from build123d import *

# Parameters (mm, degrees)
F2_DEPTH  = 25.4
F3_R      = 248.0240216894
F4_DEPTH  = 2540
F5_W      = 119.7975315154
F5_H      = 181.1522692442
F5_W_2    = 320.4690925777
F5_H_2    = 205.2030339837
F5_W_3    = 6.3688382506
F5_W_4    = 172.1075996757
F6_DEPTH  = 25.4
F7_R      = 40.7896547179
F8_DEPTH  = 2565.401
F9_R      = 164.1580524022
F10_DEPTH = 2514.6


with BuildPart() as f2:
    # F1 (on face) → F2 (new body)
    with BuildSketch(Plane.XY):
        Polygon((-21.2495476007, -69.6708932519), (-21.2495476007, 53.5316392779), (0, 53.5316392779), (0, 76.628908515), (-80.3218334913, 76.628908515), (-80.3218334913, -69.6708932519), align=None)
        Polygon((0, 76.628908515), (0, 53.5316392779), (0, -69.6708932519), (74.5332688093, -69.6708932519), (74.5332688093, 76.628908515), align=None)
        Polygon((0, -69.6708932519), (-21.2495476007, -69.6708932519), (-80.3218334913, -69.6708932519), (-80.3218334913, -80.1510289311), (74.5332688093, -80.1510289311), (74.5332688093, -69.6708932519), align=None)
    extrude(amount=F2_DEPTH)

    # F3 (on Top) → F4 (join)
    with BuildSketch(Plane.XY):
        with Locations((-47.1228808165, 30.5453538895)):
            Circle(F3_R)
    extrude(amount=-F4_DEPTH)

    # F5 (on face) → F6 (join)
    with BuildSketch(Plane.XY):
        with Locations((36.0827576369, 215.6281396747)):
            Rectangle(F5_W, F5_H)
        with Locations((-184.0505544096, 215.6281396747)):
            Rectangle(F5_W_2, F5_H)
        with Locations((-184.0505544096, 22.4504880607)):
            Rectangle(F5_W_2, F5_H_2)
        with Locations((99.1659425199, 215.6281396747)):
            Rectangle(F5_W_3, F5_H)
        Polygon((95.9815233946, -80.1510289311), (-23.8160081208, -80.1510289311), (-23.8160081208, -285.3540629148), (102.3503616452, -285.3540629148), (102.3503616452, -80.1510289311), align=None)
        with Locations((-184.0505544096, -182.752545923)):
            Rectangle(F5_W_2, F5_H_2)
        with Locations((188.404161483, 215.6281396747)):
            Rectangle(F5_W_4, F5_H)
        with Locations((188.404161483, 22.4504880607)):
            Rectangle(F5_W_4, F5_H_2)
        with Locations((188.404161483, -182.752545923)):
            Rectangle(F5_W_4, F5_H_2)
    extrude(amount=F6_DEPTH)

    # F7 (on face) → F8 (cut, through all)
    with BuildSketch(Plane.XY.offset(25.4)):
        with Locations((-161.9917303324, 89.3510133028)):
            Circle(F7_R)
    extrude(amount=-F8_DEPTH, mode=Mode.SUBTRACT)

    # F9 (on face) → F10 (cut)
    with BuildSketch(Plane.XY.offset(25.4)):
        Circle(F9_R)
    extrude(amount=-F10_DEPTH, mode=Mode.SUBTRACT)


solid = f2.part
Can you work these out from the model? Positions are in its coordinate system, mm. A direction names the side the tool comes from. Coordinates: 2 decimals unless noted, no trailing zeros. Order: outer loops, then holes, each group sorted by start corner. A loop starts at its lowest first (then second) coordinate and runs counter-clockwise, first axis right, second up. Notation, with made-up numbers: (65.5, 46.5) - (115.5, 46.5) arc R34 cw to (115.5, 83.5) - close; hole circle Ø6 at (77.5, 72.25). An arc over 180 degrees is marked (long way). Answer as a JSON object with one key per item and string values. Group by question number.
Q1. Will these pins go through, and if not, where does the flat tip stop? P1, Ø1.5, axis at x = 124, z = -2064, coming from the -Y side; P2, Ø12, axis at x = -163, z = -1143.5, coming from the -Y side; P3, Ø4, axis at y = 66, z = -1816, coming from the -X side.
Q2. We'd pull the mould along X, two halves only. Please class faces 3 (the face through (98, -183, 0)), 4 (the face through (-202.742, 91.144, -1239.342)), 5 (the face through (189.448, 105.045, -1252.22)): +X half, -X half, draft (parallel to the pull), parting line (faces both ways), or undercut.
Q3. Imagine slicing it at D-D (x = -225). Please give me the cut outline in (y, z), and give its area (3 significant figures).
Q4. I need wall thicknesses on line 1 (X direction, y = 123.5, z = -190); line 2 (Z direction, x = 184, y = -159.5); line 3 (X direction, y = 150, z = -421). Which ranges of each line are inside material? Lowest first, please. Write a range as from..to.
Q5. Imagine slicing it at A-A (x = 130). Please give me the cut outline in (y, z).
Q6. On a 3-axis mill with a long thin cutter (end or side, diameter ignored), from which of +Z, -Z, +X, -X, +Y, -Y can I reach the whole of each face in a straight line? I mean faces 1 (the face through (-2, 2, -2489.2)), 2 (the face through (-51, 34, -2540)). Say none if no direction works.
Q7. Imagine slicing it at C-C (z = -2331). Please give me the cut outline in (x, y), and give its area (3 significant figures).
Q8. Imagine slicing it at B-B (y = 0). Please give me the cut outline in (x, z).
Determined:
{
 "1": {"P1": "stops at y = -149.7", "P2": "stops at y = -191.81", "P3": "stops at x = -292.88"},
 "2": {"face 3": "draft", "face 4": "undercut", "face 5": "parting line"},
 "3": {"outline": "(-285.35, 0) - (-142.3, 0) - (-142.3, -2540) - (203.39, -2540) - (203.39, 0) - (306.2, 0) - (306.2, 25.4) - (-285.35, 25.4) - close", "area": "893,000 mm2"},
 "4": {"line 1": "x = -277.07..-184.3, -139.68..-108.15, 108.15..182.82", "line 2": "z = 0..25.4", "line 3": "x = -264.49..-66.69, 66.69..170.24"},
 "5": {"outline": "(-285.35, 0) - (-143.07, 0) - (-143.07, -2540) - (204.16, -2540) - (204.16, 0) - (306.2, 0) - (306.2, 25.4) - (100.24, 25.4) - (100.24, -2489.2) - (-100.24, -2489.2) - (-100.24, 25.4) - (-285.35, 25.4) - close"},
 "6": {"face 1": "+Z", "face 2": "-Z, +X, -X, +Y, -Y"},
 "7": {"outline": "circle Ø496.05 at (-47.12, 30.55); hole (-156.7, 48.91) arc R164.16 ccw (long way) to (-124.96, 106.45) arc R40.79 ccw (long way) to start", "area": "104,000 mm2"},
 "8": {"outline": "(-344.29, 0) - (-293.26, 0) - (-293.26, -2540) - (199.01, -2540) - (199.01, 0) - (274.46, 0) - (274.46, 25.4) - (164.16, 25.4) - (164.16, -2489.2) - (-164.16, -2489.2) - (-164.16, 25.4) - (-344.29, 25.4) - close"}
}
